Geometry check sheet. Reference: the model listing, model coordinates, mm. A direction names the side the tool comes from. Give positions to 0.01 mm unless a question says otherwise; leave off trailing zeros. Order: outer loops, then holes, each group sorted by start corner. A loop starts at its lowest first (then second) coordinate and runs counter-clockwise, first axis right, second up.
from build123d import *

# Parameters (mm, degrees)
BOSS_EXTRUDE1_DEPTH = 5.35


with BuildPart() as part:
    # Model → Boss-Extrude1 (new body)
    with BuildSketch(Plane.XY):
        with BuildLine():
            Line((5.349999992, 18.850000109), (5.349999992, 25.350000244))
            ThreePointArc((5.349999992, 25.350000244), (18.816228513, 13.067475271), (35.328051774, 5.350000109))
            Line((35.328051774, 5.350000109), (24.349999381, 5.350000109))
            Line((24.349999381, 5.350000109), (24.349999381, 0))
            Line((24.349999381, 0), (12.350000208, 0))
            Line((12.350000208, 0), (12.350000208, 5.350000109))
            Line((12.350000208, 5.350000109), (0, 5.350000109))
            Line((0, 5.350000109), (0, 18.850000109))
            Line((0, 18.850000109), (5.349999992, 18.850000109))
        make_face()
    extrude(amount=BOSS_EXTRUDE1_DEPTH)


solid = part.part
Item 1: Gauge pin test, flat ends, axial feed: pin 1 (3 mm diameter, centred on y = 20.5, z = 4.5, fed in from -X); pin 2 (1 mm diameter, centred on y = 20.5, z = 2, fed in from +X); pin 3 (1.6 mm diameter, centred on x = 4, z = 3, fed in from -Y). Record the tip position at first contact, or that the pin passes through.
Reported:
pin 1: stops at x = 5.35
pin 2: stops at x = 10.24
pin 3: stops at y = 5.35
Item 2: Sectioned sample at B-B (x = 31). Enter the section's corners in (y, z), and give its area (3 significant figures).
Reported:
outline: (5.35, 0) - (6.8, 0) - (6.8, 5.35) - (5.35, 5.35) - close
area: 7.77 mm2
Item 3: Sectioned sample at A-A (z = 1.9). Enter the section's corners in (x, y), and give its area (3 significant figures).
Reported:
outline: (0, 5.35) - (12.35, 5.35) - (12.35, 0) - (24.35, 0) - (24.35, 5.35) - (35.33, 5.35) arc R60.53 cw to (5.35, 25.35) - (5.35, 18.85) - (0, 18.85) - close
area: 370 mm2
Item 4: Scan lines: L1, parallel to Y at x = 4, z = 2.95; L2, parallel to Y at x = 32, z = 3.3; L3, parallel to X at y = 8.5, z = 1.2. Record each from-to range of solid material in increasing order.
Reported:
L1: y = 5.35 to 18.85
L2: y = 5.35 to 6.43
L3: x = 0 to 26.96
Item 5: Sectioned sample at C-C (y = 6.75). Enter the section's corners in (x, z).
Reported:
outline: (0, 0) - (31.14, 0) - (31.14, 5.35) - (0, 5.35) - close
Item 6: Set-up check for faces 1 (the flat face through (5.35, 22, 3)), 2 (the flat face through (6, 5.35, 3)), 3 (the flat face through (24.35, 3, 3)): record each of +Z, -Z, +X, -X, +Y, -Y from which the full face is reachable in a straight line by a thin tool's end or side.
Reported:
face 1: +Z, -Z, -X, +Y
face 2: +Z, -Z, -X, -Y
face 3: +Z, -Z, +X, -Y
